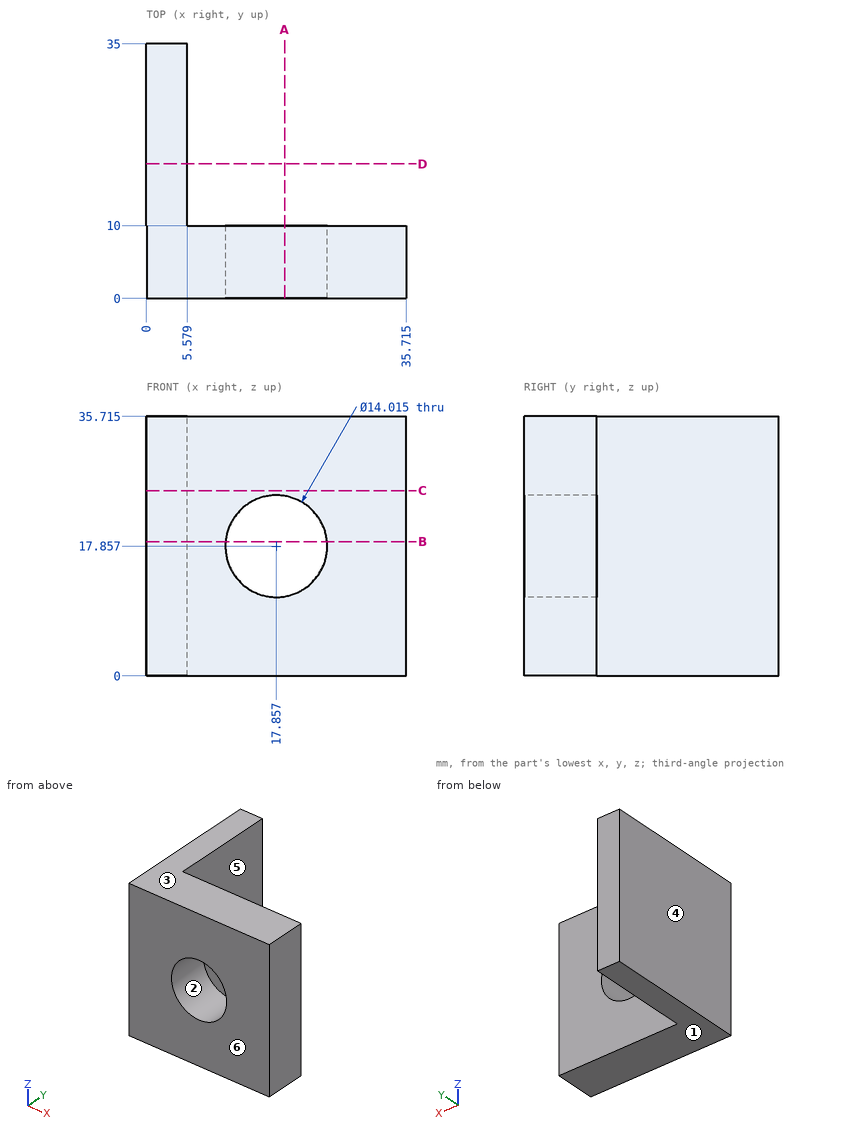
Geometry check sheet. Reference: drawing and pictorial views, mm from the part's lowest x, y, z. A direction names the side the tool comes from. Round coordinates to 2 decimals unless told otherwise and drop trailing zeros. Order: outer loops, then holes, each group sorted by start corner. A loop starts at its lowest first (then second) coordinate and runs counter-clockwise, first axis right, second up. Notation, with made-up numbers: M 32.25,7 L 54.25,7 A22 ccw 54.25,24 Z; hole C 15,-35.75 d6. An arc over 180 degrees is marked long. Write item = value, one per line.
Q1. Section check A-A (x = 19). Enter the section's corners in (y, z) (1 decimal).
Answer block:
outline = M 0,0 L 10,0 L 10,10.9 L 0,10.9 Z; M 0,24.8 L 10,24.8 L 10,35.7 L 0,35.7 Z
Q2. Section check D-D (y = 18.5). Enter the section's corners in (x, z) (1 decimal), plus the area to 3 significant figures.
Answer block:
outline = M 0,0 L 5.6,0 L 5.6,35.7 L 0,35.7 Z
area = 199 mm^2
Q3. Section check B-B (z = 18.5). Enter the section's corners in (x, y) (1 decimal).
Answer block:
outline = M 0,0 L 10.9,0 L 10.9,10 L 5.6,10 L 5.6,35 L 0,35 Z; M 24.8,0 L 35.7,0 L 35.7,10 L 24.8,10 Z
Q4. Depth check by flat-ended pin: pin 1 Ø8 at (x, z) = (28.5, 12) entering from -Y; pin 2 Ø12.5 at (y, z) = (27.5, 11.5) entering from +X; pin 3 Ø6 at (x, z) = (25, 29.5) entering from +Y. Enter the tip coordinate at first touch or a pass-through.
Answer block:
pin_1 = 0
pin_2 = 5.58
pin_3 = 10
Q5. Section check C-C (z = 25.5). Enter the section's corners in (x, y) (1 decimal).
Answer block:
outline = M 0,0 L 35.7,0 L 35.7,10 L 5.6,10 L 5.6,35 L 0,35 Z
Q6. Release check for a two-part mould opening along Z. For the marked faces 1, 2, 3 and 4 record: released by +Z, released by -Z, zero draft, split by the parting line, or undercut.
Answer block:
face_1 = released by -Z
face_2 = undercut
face_3 = released by +Z
face_4 = zero draft
Q7. Scan lines: line 1 (X direction, y = 33, z = 19); line 2 (Y direction, x = 32.5, z = 8); line 3 (X direction, y = 9.5, z = 17) (1 decimal). Record each from-to range of solid material in increasing order.
Answer block:
line_1 = 0 to 5.58
line_2 = 0 to 10
line_3 = 0 to 10.9, 24.8 to 35.7
Q8. Set-up check for the marked faces 5 and 6: record each of +Z, -Z, +X, -X, +Y, -Y from which the full face is reachable in a straight line by a thin tool's end or side.
Answer block:
face_5 = +Z, -Z, +X, +Y
face_6 = +Z, -Z, +X, -X, -Y
